```python
from build123d import *

# Parameters (mm, degrees)
BOSS_EXTRUDE1_DEPTH                     = 25
BOSS_EXTRUDE2_START                     = -25
BOSS_EXTRUDE2_DEPTH                     = 95
BOSS_EXTRUDE3_DEPTH                     = 10
CBORE_FOR_M8_HEX_HEAD_BOLT1_D           = 15
CBORE_FOR_M8_HEX_HEAD_BOLT1_CBORE_D     = 30
CBORE_FOR_M8_HEX_HEAD_BOLT1_CBORE_DEPTH = 10
CUT_EXTRUDE1_DEPTH                      = 20
BOSS_EXTRUDE4_START                     = 10
SKETCH7_R                               = 34.833333333
BOSS_EXTRUDE4_DEPTH                     = 125
BOSS_EXTRUDE5_START                     = 10
SKETCH8_R                               = 41.333333333
BOSS_EXTRUDE5_DEPTH                     = 125
CUT_EXTRUDE2_REACH                      = 315.988
SKETCH9_R                               = 20.5
CUT_EXTRUDE3_REACH                      = 322.331
SKETCH10_R                              = 20.5
CHAMFER1_SIZE                           = 2


with BuildPart() as part:
    # Sketch1 → Boss-Extrude1 (new body)
    with BuildSketch(Plane(origin=(0, 0, 0), x_dir=(1, 0, 0), z_dir=(0, 1, 0))):
        with BuildLine():
            Line((-39, 40), (159, 40))
            ThreePointArc((159, 40), (166.071067812, 37.071067812), (169, 30))
            Line((169, 30), (169, -159))
            ThreePointArc((169, -159), (166.071067812, -166.071067812), (159, -169))
            Line((159, -169), (-39, -169))
            ThreePointArc((-39, -169), (-46.071067812, -166.071067812), (-49, -159))
            Line((-49, -159), (-49, 30))
            ThreePointArc((-49, 30), (-46.071067812, 37.071067812), (-39, 40))
        make_face()
    extrude(amount=BOSS_EXTRUDE1_DEPTH)

    # Sketch2 → Boss-Extrude2 (add)
    with BuildSketch(Plane(origin=(0, 25, 0), x_dir=(1, 0, 0), z_dir=(0, 1, 0)).offset(BOSS_EXTRUDE2_START)):
        with BuildLine():
            Line((0, -89), (0, -169))
            Line((0, -169), (15, -169))
            Line((15, -169), (15, -102.912584265))
            ThreePointArc((15, -102.912584265), (73.539105243, -73.539105243), (102.912584265, -15))
            Line((102.912584265, -15), (169, -15))
            Line((169, -15), (169, 0))
            Line((169, 0), (89, 0))
            ThreePointArc((89, 0), (62.932503526, -62.932503526), (0, -89))
        make_face()
    extrude(amount=BOSS_EXTRUDE2_DEPTH)

    # Sketch3 → Boss-Extrude3 (add)
    with BuildSketch(Plane(origin=(0, 25, 0), x_dir=(1, 0, 0), z_dir=(0, 1, 0))):
        with BuildLine():
            Line((124, -109), (169, -109))
            Line((169, -109), (169, -159))
            ThreePointArc((169, -159), (166.071067812, -166.071067812), (159, -169))
            Line((159, -169), (109, -169))
            Line((109, -169), (109, -124))
            ThreePointArc((109, -124), (113.393398282, -113.393398282), (124, -109))
        make_face()
    extrude(amount=BOSS_EXTRUDE3_DEPTH)

    # CBORE for M8 Hex Head Bolt1 (through all)
    with Locations(Plane(origin=(0, 35, 0), x_dir=(1, 0, 0), z_dir=(0, 1, 0))):
        with Locations((139, -139)):
            CounterBoreHole(CBORE_FOR_M8_HEX_HEAD_BOLT1_D / 2, CBORE_FOR_M8_HEX_HEAD_BOLT1_CBORE_D / 2, CBORE_FOR_M8_HEX_HEAD_BOLT1_CBORE_DEPTH)

    # Sketch6 → Cut-Extrude1 (cut)
    with BuildSketch(Plane(origin=(0, 25, 0), x_dir=(1, 0, 0), z_dir=(0, 1, 0))):
        with BuildLine():
            Line((100, -150), (100, -124))
            ThreePointArc((100, -124), (107.029437252, -107.029437252), (124, -100))
            Line((124, -100), (150, -100))
            ThreePointArc((150, -100), (157.071067812, -97.071067812), (160, -90))
            Line((160, -90), (160, -34))
            ThreePointArc((160, -34), (157.071067812, -26.928932188), (150, -24))
            Line((150, -24), (118.207444774, -24))
            ThreePointArc((118.207444774, -24), (112.192558093, -26.011186683), (108.59708341, -31.235772358))
            ThreePointArc((108.59708341, -31.235772358), (79.903066274, -79.903066274), (31.235772358, -108.59708341))
            ThreePointArc((31.235772358, -108.59708341), (26.011186683, -112.192558093), (24, -118.207444774))
            Line((24, -118.207444774), (24, -150))
            ThreePointArc((24, -150), (26.928932188, -157.071067812), (34, -160))
            Line((34, -160), (90, -160))
            ThreePointArc((90, -160), (97.071067812, -157.071067812), (100, -150))
        make_face()
    extrude(amount=-CUT_EXTRUDE1_DEPTH, mode=Mode.SUBTRACT)

    # Sketch7 → Boss-Extrude4 (add)
    with BuildSketch(Plane.XY.offset(169).offset(BOSS_EXTRUDE4_START)):
        with Locations((7.5, 95)):
            Circle(SKETCH7_R)
    extrude(amount=-BOSS_EXTRUDE4_DEPTH)

    # Sketch8 → Boss-Extrude5 (add)
    with BuildSketch(Plane(origin=(169, 0, 0), x_dir=(0, 0, -1), z_dir=(1, 0, 0)).offset(BOSS_EXTRUDE5_START)):
        with Locations((-7.5, 95)):
            Circle(SKETCH8_R)
    extrude(amount=-BOSS_EXTRUDE5_DEPTH)

    # Sketch9 → Cut-Extrude2 (cut, up to next)
    with BuildSketch(Plane.XY.offset(179), mode=Mode.PRIVATE) as cut_extrude2_sk1:
        with Locations((7.5, 95)):
            Circle(SKETCH9_R)
    cut_extrude2_tool1 = extrude(cut_extrude2_sk1.sketch, amount=-CUT_EXTRUDE2_REACH, mode=Mode.PRIVATE) & part.part
    add(cut_extrude2_tool1.solids().sort_by_distance((7.5, 95, 179))[0], mode=Mode.SUBTRACT)

    # Sketch10 → Cut-Extrude3 (cut, up to next)
    with BuildSketch(Plane(origin=(179, 0, 0), x_dir=(0, 0, -1), z_dir=(1, 0, 0)), mode=Mode.PRIVATE) as cut_extrude3_sk1:
        with Locations((-7.5, 95)):
            Circle(SKETCH10_R)
    cut_extrude3_tool1 = extrude(cut_extrude3_sk1.sketch, amount=-CUT_EXTRUDE3_REACH, mode=Mode.PRIVATE) & part.part
    add(cut_extrude3_tool1.solids().sort_by_distance((179, 95, 7.5))[0], mode=Mode.SUBTRACT)

    # Chamfer1
    chamfer1_edges = [part.edges().sort_by_distance(p)[0] for p in [
        (-13, 95, 179),
        (-13, 95, 54),
        (179, 95, 28),
        (54, 95, 28),
    ]]
    chamfer(chamfer1_edges, length=CHAMFER1_SIZE)


solid = part.part
```
CAD build for the part. Positions are in the model's coordinates, mm. A direction names the side the tool comes from. Round coordinates to 2 decimals unless told otherwise and drop trailing zeros. Write each loop counter-clockwise with the first axis right and the second up, starting at its lowest first coordinate (ties: lowest second). Pieces come first, ordered by that corner, then holes. Notation, with made-up numbers: (-3, 56.25) - (49, 56.25) arc R17 cw to (49, 85.25) - close; hole circle Ø7 at (-27, -11). An arc over 180 degrees is marked (long way). Return JSON: item names as keys, results as strings. Group by question number.
Item 1: Flat gauge pins, fed straight in: pin 1 Ø6 at (y, z) = (110.5, 61.5) entering from -X; pin 2 Ø10 at (x, y) = (58, 49.5) entering from +Z; pin 3 Ø16 at (x, y) = (135.5, 17.5) entering from +Z. Where does each tip first touch, or does it go through?
Item 2: Probe probe 1 along X at (y, z) = (29.5, 139); probe 2 along Y at (x, z) = (87, 7). List the from-to ranges inside material, lowest first.
Item 3: Band-saw the part on A-A on z = 139. List the corners of the cut face in (x, y), plus the area to 3 significant figures.
Item 4: Band-saw the part on B-B on x = 139. List the corners of the cut face in (y, z), plus the area to 3 significant figures.
Item 5: Band-saw the part on C-C on y = 31. List the corners of the cut face in (x, z), plus the area to 3 significant figures.
Item 6: Band-saw the part on D-D on z = 7.5. List the corners of the cut face in (x, y).
Item 7: Mould opens along Y. For faces 4 (the face through (67, 95, 72)), 5 (the face through (91, 5, 91)), 6 (the face through (157.15, 15.14, 27.01)), 7 (the face through (131.846, 12.325, 136.747)) say: +Y half, -Y half, draft (parallel to the pull), parting line (faces both ways), or undercut.
Item 8: 3-axis set-ups, long thin cutter, end or side, ignore diameter. For faces 1 (the face through (26.066, 15.14, 112.121)), 2 (the face through (165.99, 12.32, -37.15)), 3 (the face through (96.99, 15.14, 157.15)): which of +Z, -Z, +X, -X, +Y, -Y reach the whole face in a straight line?
Resolved:
{
 "1": {"pin 1": "stops at x = -25.01", "pin 2": "stops at z = 89.48", "pin 3": "stops at z = 169"},
 "2": {"probe 1": "x = 0 to 15, 109 to 124, 154 to 169", "probe 2": "y = 0 to 25, 53.67 to 74.51, 115.49 to 136.33"},
 "3": {"outline": "(-49, 0) - (131.5, 0) - (131.5, 25) - (124, 25) - (124, 35) - (109, 35) - (109, 25) - (100, 25) - (100, 5) - (24, 5) - (24, 25) - (15, 25) - (15, 60.98) arc R34.83 ccw (long way) to (0, 60.98) - (0, 25) - (-49, 25) - close; (146.5, 0) - (169, 0) - (169, 35) - (154, 35) - (154, 25) - (146.5, 25) - close; hole circle Ø41 at (7.5, 95)", "area": "6,880 mm²"},
 "4": {"outline": "(0, -40) - (25, -40) - (25, 0) - (54.35, 0) arc R41.33 ccw (long way) to (54.35, 15) - (25, 15) - (25, 24) - (5, 24) - (5, 100) - (25, 100) - (25, 109) - (35, 109) - (35, 124) - (25, 124) - (25, 131.5) - (0, 131.5) - close; (0, 146.5) - (25, 146.5) - (25, 154) - (35, 154) - (35, 169) - (0, 169) - close; hole circle Ø41 at (95, 7.5)", "area": "8,110 mm²"},
 "5": {"outline": "(0, 89) arc R89 cw to (89, 0) - (169, 0) - (169, 15) - (102.91, 15) arc R104 ccw to (15, 102.91) - (15, 169) - (0, 169) - close; (109, 124) arc R15 ccw to (124, 109) - (169, 109) - (169, 159) arc R10 ccw to (159, 169) - (109, 169) - close; hole circle Ø30 at (139, 139)", "area": "7,060 mm²"},
 "6": {"outline": "(-49, 0) - (169, 0) - (169, 53.67) - (179, 53.67) - (179, 72.5) - (177, 74.5) - (56, 74.5) - (54, 72.5) - (54, 53.67) - (88.68, 53.67) - (88.68, 25) - (-49, 25) - close; (54, 117.5) - (56, 115.5) - (177, 115.5) - (179, 117.5) - (179, 136.33) - (54, 136.33) - close"},
 "7": {"face 4": "+Y half", "face 5": "undercut", "face 6": "undercut", "face 7": "draft"},
 "8": {"face 1": "none", "face 2": "-Z, +X, -Y", "face 3": "+Y"}
}
